The model under review builds one solid part; all positions refer to its coordinate system, in mm. Coordinates: 2 decimals unless noted, no trailing zeros. Write each loop counter-clockwise with the first axis right and the second up, starting at its lowest first coordinate (ties: lowest second). Pieces come first, ordered by that corner, then holes. Notation, with made-up numbers: M 89,66 L 112,66 A13 ccw 112,79 Z; hole C -39.75,38.25 d7. An arc over 180 degrees is marked long. Answer as a JSON object with one key per item and string values.
Autodesk Inventor part; units mm, degrees
ref_plane "YZ Plane" through (0, 0, 0) normal (1, 0, 0) x (0, 1, 0)
ref_plane "XZ Plane" through (0, 0, 0) normal (0, 1, 0) x (-1, 0, 0)
ref_plane "XY Plane" through (0, 0, 0) normal (0, 0, 1) x (1, 0, 0)
sketch "Sketch1" plane through (0, 0, 0) normal (1, 0, 0) x (0, 1, 0)
  circle A0 centre (1.9588, 3.377) radius 2.2698
  circle A1 centre (1.9588, 3.377) radius 2.2698
  line L0 (1.9588, 3.377) -> (1.9588, 0)
  line L1 (1.9588, 0) -> (0, 0)
  line L2 (0, 0) -> (0, 3.377)
  line L3 (0, 3.377) -> (1.9588, 3.377)
  circle A2 centre (3.3027, -3.8845) radius 2.2698
  line L4 (0, 0) -> (0, -3.8845)
  line L5 (0, -3.8845) -> (3.3027, -3.8845)
  line L6 (3.3027, -3.8845) -> (3.3027, 0)
  line L7 (3.3027, 0) -> (0, 0)
  circle A3 centre (0, 0) radius 13.5
  dimension "d0" = 4.5396
  dimension "d1" = 3.377
  dimension "d2" = 1.9588
  dimension "d3" = 3.8845
  dimension "d4" = 3.3026
  dimension "d5" = 4.5396
  dimension "d6" = 27
extrude "Extrusion1" add sketch "Sketch1" along normal blind 0.95 contours A0 L0 L1 L2 | L1 L7 L6 A2 L5 L4 | A3
sketch "Sketch2" plane through (0.95, 0, 0) normal (1, 0, 0) x (0, 0, -1)
  circle A0 centre (-3.377, 1.9588) radius 2.2698
  circle A1 centre (-3.377, 1.9588) radius 2.5
  circle A2 centre (3.8845, 3.3027) radius 2.2698
  circle A3 centre (3.8845, 3.3027) radius 2.5
  point P0 (0, 0)
  dimension "d9" = 5
  dimension "d10" = 5
extrude "Extrusion2" cut sketch "Sketch2" against normal blind 0.95 contours A0 | A1 | A2 | A3
fillet "Fillet1" radius 0.1 5 edges at (0.95, 1.9588, 5.877) (0.95, 3.3027, -1.3845) (0, 3.3027, -1.3845) (0, 1.9588, 5.877) (0, -13.5, 0)
chamfer "Chamfer1" distance 0.2 angle 45 1 edges at (0.95, -13.5, 0)
properties part number "PlateGantryMountSymbolDisc"
(1) For pin 1 Ø3 at (y, z) = (3.3, -3.88) entering from +X, flat-tipped, find the tip position at first contact; note if it passes through.
Results list:
{"pin 1": "through"}
(2) Wall thickness on line 1 along Z through (x, y) = (0.55, 0.5); line 2 along Y through (x, z) = (0.15, 1.75); line 3 along Y through (x, z) = (0.15, 4.5): over which ranges is each line inside the solid? List them lowest first. Write a range as from..to.
Results list:
{"line 1": "-13.49..1.35, 5.41..13.49", "line 2": "-13.39..0.06, 3.86..13.39", "line 3": "-12.73..-0.27, 4.19..12.73"}
(3) Draft analysis for pull direction Z (two halves, no side actions). For faces 1 (the face through (0.48, 4.438, 3.702)), 2 (the face through (0, 0, 0)), 3 (the face through (0.42, -2.93, 13.18)), state which applies: released by +Z, released by -Z, zero draft, split by the parting line, or undercut.
Results list:
{"face 1": "undercut", "face 2": "zero draft", "face 3": "split by the parting line"}
(4) Add section A-A on x = 0.45. Give the boundary of the cut face in (y, z), and give its area (3 significant figures).
Results list:
{"outline": "C 0,0 d27; hole C 1.96,3.38 d5; hole C 3.3,-3.88 d5", "area": "533 mm²"}
